```python
from build123d import *

# Parameters (mm, degrees)
SKETCH1_R           = 28.575
BOSS_EXTRUDE1_DEPTH = 530
SKETCH2_OUTSIDE_W   = 166.376
SKETCH2_OUTSIDE_H   = 166.376
SKETCH2_OUTSIDE_R   = 18.9
CUT_EXTRUDE1_DEPTH  = 38
SKETCH3_OUTSIDE_W   = 166.376
SKETCH3_OUTSIDE_H   = 166.376
SKETCH3_OUTSIDE_R   = 20.64
CUT_EXTRUDE2_DEPTH  = 40
SKETCH4_OUTSIDE_W   = 166.376
SKETCH4_OUTSIDE_H   = 166.376
SKETCH4_OUTSIDE_R   = 24.5
CUT_EXTRUDE3_DEPTH  = 55
SKETCH5_R           = 5
BOSS_EXTRUDE2_DEPTH = 5
CHAMFER1_SIZE       = 1


with BuildPart() as part:
    # Sketch1 → Boss-Extrude1 (new body)
    with BuildSketch(Plane.XY):
        Circle(SKETCH1_R)
    extrude(amount=BOSS_EXTRUDE1_DEPTH)

    # Sketch2 outside → Cut-Extrude1 (cut)
    with BuildSketch(Plane.XY.offset(530)):
        Rectangle(SKETCH2_OUTSIDE_W, SKETCH2_OUTSIDE_H)
        Circle(SKETCH2_OUTSIDE_R, mode=Mode.SUBTRACT)
    extrude(amount=-CUT_EXTRUDE1_DEPTH, mode=Mode.SUBTRACT)

    # Sketch3 outside → Cut-Extrude2 (cut)
    with BuildSketch(Plane.XY.offset(492)):
        Rectangle(SKETCH3_OUTSIDE_W, SKETCH3_OUTSIDE_H)
        Circle(SKETCH3_OUTSIDE_R, mode=Mode.SUBTRACT)
    extrude(amount=-CUT_EXTRUDE2_DEPTH, mode=Mode.SUBTRACT)

    # Sketch4 outside → Cut-Extrude3 (cut)
    with BuildSketch(Plane.XY.offset(452)):
        Rectangle(SKETCH4_OUTSIDE_W, SKETCH4_OUTSIDE_H)
        Circle(SKETCH4_OUTSIDE_R, mode=Mode.SUBTRACT)
    extrude(amount=-CUT_EXTRUDE3_DEPTH, mode=Mode.SUBTRACT)

    # Sketch5 → Boss-Extrude2 (add)
    with BuildSketch(Plane(origin=(0, 0, 0), x_dir=(-1, 0, 0), z_dir=(0, 0, -1))):
        Circle(SKETCH5_R)
    extrude(amount=BOSS_EXTRUDE2_DEPTH)

    # Chamfer1
    chamfer1_edges = [part.edges().sort_by_distance(p)[0] for p in [
        (-18.9, 0, 530),
        (-28.575, 0, 397),
        (-24.5, 0, 452),
    ]]
    chamfer(chamfer1_edges, length=CHAMFER1_SIZE)


solid = part.part
```
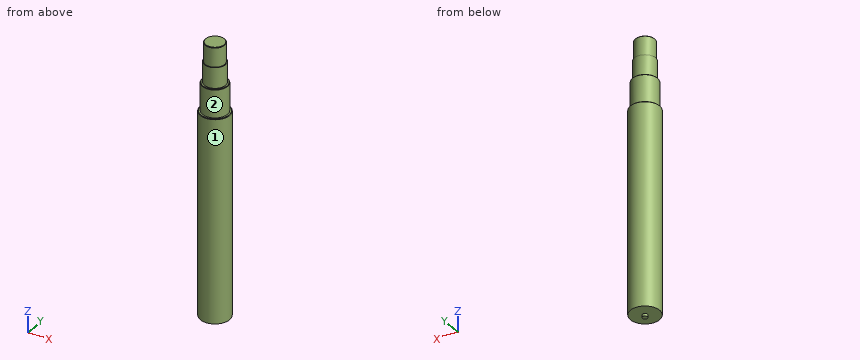
Work out the finished part from the listing and answer in its coordinate system (mm). Face numbers are marked on the shaded views. A direction names the side the tool comes from. Give positions to 0.01 mm unless a question says otherwise; leave off trailing zeros. Order: outer loops, then holes, each group sorted by start corner. A loop starts at its lowest first (then second) coordinate and runs counter-clockwise, first axis right, second up. Notation, with made-up numbers: (32.25, 35) -> (82.25, 35) arc R20 ccw to (82.25, 49) -> close; hole circle Ø10 at (-15, 85.5). An arc over 180 degrees is marked (long way). Answer as CSV lines item,"result". Start each with the question number.
(1) Consider line 1 along Z through (x, y) = (4.5, 16); line 2 along Z through (x, y) = (-3, 26); line 3 along X through (y, z) = (21, 228.5). Determine where each line is inside the solid, lowest interval first.
(2) Each of these flat-tipped pins is pushed along its axis until it touches: pin 1 Ø8 at (x, z) = (2.5, 126.5) entering from +Y (3 decimals); pin 2 Ø6 at (x, y) = (-3, -17.5) entering from -Z; pin 3 Ø3 at (y, z) = (6, 369.5) entering from -X. Where does it stop, or does it pass through?
(3) Section A-A, the plane y = 0 is taken. Write down the section's boundary in (x, z) (3 decimals).
(4) Which of the six approach directions +Z, -Z, +X, -X, +Y, -Y give full straight-line access (tool end or side, diameter ignored) to the marked faces 1 and 2?
(5) Section C-C, the plane z = 74 is taken. Write down the section's boundary in (x, y) (3 decimals), plus the area to 3 significant figures.
Entries:
1,line 1,"0 to 530"
1,line 2,"0 to 397"
1,line 3,"-19.38 to 19.38"
2,pin 1,"y = 28.575"
2,pin 2,"z = 0"
2,pin 3,"x = -28.22"
3,outline,"(-28.575, 0) -> (-5, 0) -> (-5, -5) -> (5, -5) -> (5, 0) -> (28.575, 0) -> (28.575, 396) -> (27.575, 397) -> (24.5, 397) -> (24.5, 451) -> (23.5, 452) -> (20.64, 452) -> (20.64, 492) -> (18.9, 492) -> (18.9, 529) -> (17.9, 530) -> (-17.9, 530) -> (-18.9, 529) -> (-18.9, 492) -> (-20.64, 492) -> (-20.64, 452) -> (-23.5, 452) -> (-24.5, 451) -> (-24.5, 397) -> (-27.575, 397) -> (-28.575, 396) -> close"
4,face 1,"+Z, -Z"
4,face 2,"+Z"
5,outline,"circle Ø57.15 at (0, 0)"
5,area,"2,570 mm²"
